For this review, take the finished solid that the model builds, in its own axes (mm). A direction names the side the tool comes from. Give positions to 0.01 mm unless a question says otherwise; leave off trailing zeros. Write each loop counter-clockwise with the first axis right and the second up, starting at its lowest first coordinate (ties: lowest second). Pieces come first, ordered by that corner, then holes.
1) Machinability: for faces 1 (the face through (-5, 1, 2)), 2 (the face through (5.75, -8, 1.7)), 3 (the face through (0, 28.761, 3)), which of the approach directions +Z, -Z, +X, -X, +Y, -Y give a long, thin tool a straight path to every point of the face, cutting with its end or side? Answer none if there is none.
2) We need section A-A on z = 3. Give the boundary of the cut face in (x, y).
3) We need section C-C on x = 0.25. Give the boundary of the cut face in (y, z), and give its area (3 significant figures).
4) We need section D-D on x = 4.25. Give the boundary of the cut face in (y, z), and give its area (3 significant figures).
5) Wall thickness on line 1 along Y through (x, z) = (0, 2); line 2 along X through (y, z) = (-7, 1); line 3 along Z through (x, y) = (-2.25, -22.5): over which ranges is each line inside the solid? List them lowest first.
6) Draft analysis for pull direction Y (two halves, no side actions). For faces 4 (the face through (0, -30, 6.4)), 5 (the face through (4, 1, 2)), 6 (the face through (-4.25, 0, 1)), 7 (the face through (0, -31.639, 3)), state which applies: pulls with the +Y half, pulls with the -Y half, needs draft (parallel to the pull), parting line crosses it, or undercut.
7) We need section B-B on y = 16. Give the boundary of the cut face in (x, z).
8) For P1, Ø0.8, axis at x = -5, y = 9, coming from the +Z side; P2, Ø5, axis at x = -0.5, y = 7.5, coming from the +Z side, all flat-tipped, find the tip position at first contact; note any pin that passes through.
from build123d import *

# Parameters (mm, degrees)
F0_W     = 11.5
F0_H     = 62
F1_DEPTH = 2
F2_W     = 7.5
F2_H     = 57
F3_DEPTH = 1.5
F4_W     = 6
F4_H     = 20
F5_DEPTH = 0.5
F6_W     = 11.5
F6_H     = 3.4
F6_H_2   = 1.6
F7_DEPTH = 4.4


with BuildPart() as f1:
    # F0 (on Top) → F1 (new body)
    with BuildSketch(Plane.XY):
        with Locations((0, -0.639212)):
            Rectangle(F0_W, F0_H)
    extrude(amount=F1_DEPTH)

    # F2 (on face) → F3 (cut)
    with BuildSketch(Plane.XY.offset(2)):
        with Locations((-0.5, 0.260788)):
            Rectangle(F2_W, F2_H)
    extrude(amount=-F3_DEPTH, mode=Mode.SUBTRACT)

    # F4 (on face) → F5 (cut, through all)
    with BuildSketch(Plane.XY.offset(0.5)):
        with Locations((-0.75, 8.760788)):
            Rectangle(F4_W, F4_H)
    extrude(amount=-F5_DEPTH, mode=Mode.SUBTRACT)

    # F6 (on face) → F7 (join)
    with BuildSketch(Plane.XY.offset(2)):
        with Locations((0, -29.939212)):
            Rectangle(F6_W, F6_H)
        with Locations((0, 29.560788)):
            Rectangle(F6_W, F6_H_2)
    extrude(amount=F7_DEPTH)


solid = f1.part
Results list:
1. face 1: +Z, +X, -X
1. face 2: +Z, -Z, +X, +Y, -Y
1. face 3: +Z
2. outline: (-5.75, -31.64) - (5.75, -31.64) - (5.75, -28.24) - (-5.75, -28.24) - close; (-5.75, 28.76) - (5.75, 28.76) - (5.75, 30.36) - (-5.75, 30.36) - close
3. outline: (-31.64, 0) - (-1.24, 0) - (-1.24, 0.5) - (-28.24, 0.5) - (-28.24, 6.4) - (-31.64, 6.4) - close; (18.76, 0) - (30.36, 0) - (30.36, 6.4) - (28.76, 6.4) - (28.76, 0.5) - (18.76, 0.5) - close
3. area: 50.5 mm2
4. outline: (-31.64, 0) - (30.36, 0) - (30.36, 6.4) - (28.76, 6.4) - (28.76, 2) - (-28.24, 2) - (-28.24, 6.4) - (-31.64, 6.4) - close
4. area: 146 mm2
5. line 1: y = -31.64 to -28.24, 28.76 to 30.36
5. line 2: x = -5.75 to -4.25, 3.25 to 5.75
5. line 3: z = 0 to 0.5
6. face 4: needs draft
6. face 5: undercut
6. face 6: undercut
6. face 7: pulls with the -Y half
7. outline: (-5.75, 0) - (-3.75, 0) - (-3.75, 0.5) - (-4.25, 0.5) - (-4.25, 2) - (-5.75, 2) - close; (2.25, 0) - (5.75, 0) - (5.75, 2) - (3.25, 2) - (3.25, 0.5) - (2.25, 0.5) - close
8. P1: stops at z = 2
8. P2: passes through
